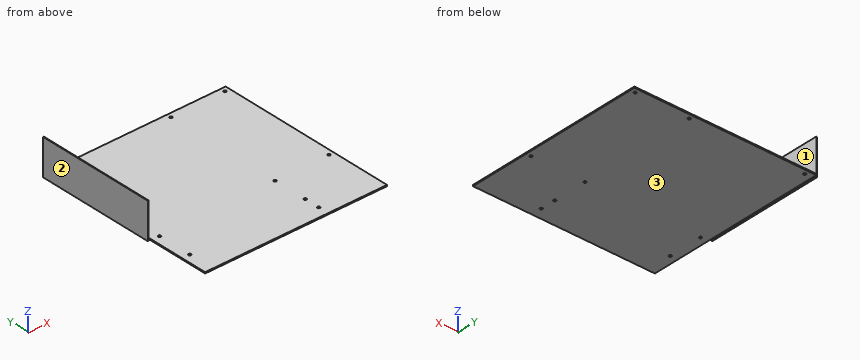
from build123d import *

# Parameters (mm, degrees)
SKETCH_1_W           = 244
SKETCH_1_H           = 244
EXTRUDE_1_DEPTH      = 1.6
SKETCH_2_R           = 1.75
CUT_EXTRUDE_1_DEPTH  = 346.071818612
EXTRUDE_2_DEPTH      = 44.45
EXTRUDE_2_DEPTH_BACK = 3.81
SKETCH_3_W           = 1
SKETCH_3_H           = 158.75


with BuildPart() as part:
    # 草图1 → 凸台-拉伸1 (new body)
    with BuildSketch(Plane.XY):
        with Locations((122, 122)):
            Rectangle(SKETCH_1_W, SKETCH_1_H)
    extrude(amount=EXTRUDE_1_DEPTH)

    # 草图2 → 切除-拉伸1 (cut, through all)
    with BuildSketch(Plane.XY.offset(1.6)):
        with Locations((10.16, 34.63)):
            Circle(SKETCH_2_R)
        with Locations((10.16, 80.35)):
            Circle(SKETCH_2_R)
        with Locations((165.1, 34.63)):
            Circle(SKETCH_2_R)
        with Locations((165.1, 80.35)):
            Circle(SKETCH_2_R)
        with Locations((165.1, 14.31)):
            Circle(SKETCH_2_R)
        with Locations((237.49, 80.35)):
            Circle(SKETCH_2_R)
        with Locations((10.16, 237.83)):
            Circle(SKETCH_2_R)
        with Locations((165.1, 237.83)):
            Circle(SKETCH_2_R)
        with Locations((237.49, 237.83)):
            Circle(SKETCH_2_R)
    extrude(amount=-CUT_EXTRUDE_1_DEPTH, mode=Mode.SUBTRACT)

    # 草图3 → 凸台-拉伸2 (add, two sides: drawn at the far end of the back side and taken through both)
    with BuildSketch(Plane.XY.offset(1.6).offset(-EXTRUDE_2_DEPTH_BACK)):
        with Locations((-0.5, 164.625)):
            Rectangle(SKETCH_3_W, SKETCH_3_H)
    extrude(amount=EXTRUDE_2_DEPTH + EXTRUDE_2_DEPTH_BACK)


solid = part.part
Verification items for the finished model (mm, model axes). Face numbers are marked on the shaded views. A direction names the side the tool comes from. Coordinates: 2 decimals unless noted, no trailing zeros. Write each loop counter-clockwise with the first axis right and the second up, starting at its lowest first coordinate (ties: lowest second). Pieces come first, ordered by that corner, then holes. Notation, with made-up numbers: (66.5, 31.25) -> (86.5, 31.25) arc R33 ccw to (86.5, 67.25) -> close; hole circle Ø7 at (81.25, 32). An arc over 180 degrees is marked (long way). One line per item, written item: value. Start each with the question number.
Q1. Cross-section at A-A on y = 70. Enter the section's corners in (x, z).
Q2. Go/stop test with flat-tipped pins: P1, Ø10, axis at y = 169, z = 15.5, coming from the +X side; P2, Ø5, axis at x = 186.5, y = 154, coming from the +Z side; P3, Ø3, axis at x = 10.16, y = 237.83, coming from the +Z side; P4, Ø1.8, axis at y = 32.5, z = 0.5, coming from the -X side. Record where each tip stops, or that it passes through.
Q3. Access from +Z, -Z, +X, -X, +Y, -Y to the whole of each face (thin tool, end or side, straight path). Record for the marked faces 1, 2 and 3.
Q4. Thickness scan on L1, parallel to Y at x = 10.16, z = 0.6; L2, parallel to X at y = 237.83, z = 1.3; L3, parallel to X at y = 80, z = 1. Record the ranges inside material, lowest first. Write a range as from..to.
Checked values:
1. outline: (0, 0) -> (244, 0) -> (244, 1.6) -> (0, 1.6) -> close
2. P1: stops at x = 0
2. P2: stops at z = 1.6
2. P3: passes through
2. P4: stops at x = 0
3. face 1: +Z, +X, +Y, -Y
3. face 2: +Z, -Z, -X, +Y, -Y
3. face 3: -Z, +X, +Y, -Y
4. L1: y = 0..32.88, 36.38..78.6, 82.1..236.08, 239.58..244
4. L2: x = -1..8.41, 11.91..163.35, 166.85..235.74, 239.24..244
4. L3: x = 0..8.45, 11.87..163.39, 166.81..235.78, 239.2..244
